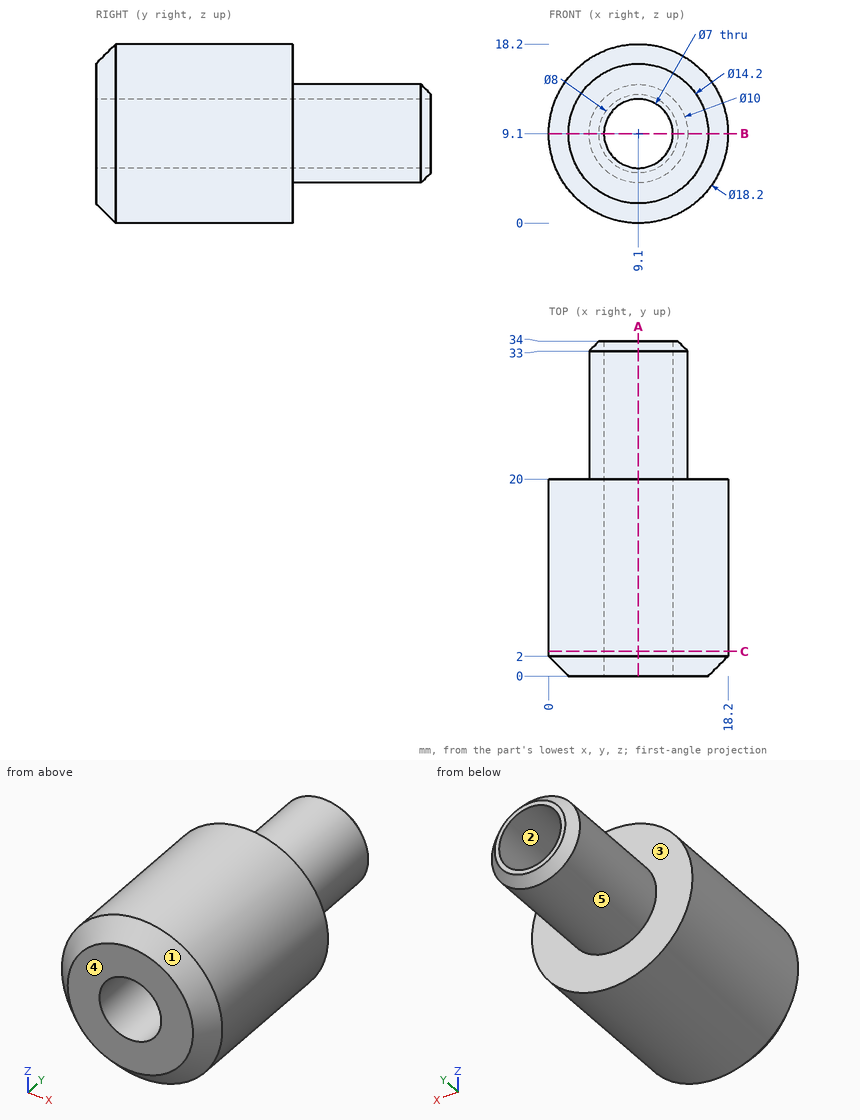
Here's the drawing with two shaded views (mm, measured from the low corner). I have some questions. A direction names the side the tool comes from. Coordinates: 2 decimals unless noted, no trailing zeros. Write each loop counter-clockwise with the first axis right and the second up, starting at its lowest first coordinate (ties: lowest second). Pieces come first, ordered by that corner, then holes. Notation, with made-up numbers: (6.25, -16) -> (33.25, -16) arc R12 cw to (33.25, -6) -> close; hole circle Ø8 at (48, 39). An arc over 180 degrees is marked (long way). Use a Markdown table: item, result. Add a question column.
(1) If we section it at C-C, the plane y = 2.5: Write out the boundary of the cut face in (x, z), and give its area (3 significant figures).
(2) For the marked faces 4 and 5, which set-ups out of +Z, -Z, +X, -X, +Y, -Y let a thin tool reach every point of the face, with its end or its side?
(3) We'd pull the mould along X, two halves only. Please class the marked faces 1, 2 and 3: +X half, -X half, draft (parallel to the pull), parting line (faces both ways), or undercut.
(4) If we section it at A-A, the plane x = 9.1: Write out the boundary of the cut face in (y, z).
(5) I'm going to push flat-ended pins straight in: P1, Ø2, axis at y = 18.5, z = 13, coming from the +X side; P2, Ø1.5, axis at y = 14, z = 4.5, coming from the +X side; P3, Ø1.5, axis at y = 7.5, z = 5, coming from the -X side. Where does each tip first touch, or does it pass through?
(6) Please list where these lines run through material, in increasing order: line 1 (Z direction, x = 9.1, y = 15.5); line 2 (X direction, y = 23.5, z = 9.1); line 3 (Y direction, x = 4.5, z = 7).
(7) If we section it at B-B, the plane z = 9.1: Write out the boundary of the cut face in (x, y).
Outcome:
| question | item | result |
|---|---|---|
| 1 | outline | circle Ø18.2 at (9.1, 9.1); hole circle Ø7 at (9.1, 9.1) |
| 1 | area | 222 mm^2 |
| 2 | face 4 | +Z, -Z, +X, -X, -Y |
| 2 | face 5 | +Y |
| 3 | face 1 | parting line |
| 3 | face 2 | undercut |
| 3 | face 3 | draft |
| 4 | outline | (0, 2) -> (2, 0) -> (20, 0) -> (20, 4.1) -> (33, 4.1) -> (34, 5.1) -> (34, 5.6) -> (0, 5.6) -> close; (0, 12.6) -> (34, 12.6) -> (34, 13.1) -> (33, 14.1) -> (20, 14.1) -> (20, 18.2) -> (2, 18.2) -> (0, 16.2) -> close |
| 5 | P1 | stops at x = 17.73 |
| 5 | P2 | stops at x = 17.35 |
| 5 | P3 | stops at x = 0.64 |
| 6 | line 1 | z = 0 to 5.6, 12.6 to 18.2 |
| 6 | line 2 | x = 4.1 to 5.6, 12.6 to 14.1 |
| 6 | line 3 | y = 0 to 20 |
| 7 | outline | (0, 2) -> (2, 0) -> (5.6, 0) -> (5.6, 34) -> (5.1, 34) -> (4.1, 33) -> (4.1, 20) -> (0, 20) -> close; (12.6, 0) -> (16.2, 0) -> (18.2, 2) -> (18.2, 20) -> (14.1, 20) -> (14.1, 33) -> (13.1, 34) -> (12.6, 34) -> close |
